```python
from build123d import *

# Parameters (mm, degrees)
CROQUIS1_W                = 7
CROQUIS1_H                = 18
SALIENTE_EXTRUIR1_DEPTH   = 9
SALIENTE_EXTRUIR1_2_DEPTH = 9
SALIENTE_EXTRUIR1_3_DEPTH = 9
SALIENTE_EXTRUIR1_4_DEPTH = 9
SALIENTE_EXTRUIR1_5_DEPTH = 9
SALIENTE_EXTRUIR1_6_DEPTH = 9
CROQUIS2_W                = 48.25
CROQUIS2_H                = 4
SALIENTE_EXTRUIR2_DEPTH   = 9
CROQUIS3_R                = 2.5
CROQUIS3_R_2              = 2
SALIENTE_EXTRUIR3_DEPTH   = 5.5
CROQUIS4_R                = 1
CORTAR_EXTRUIR1_DEPTH     = 53.278700252
CROQUIS5_W                = 6
CROQUIS5_H                = 8
CORTAR_EXTRUIR2_DEPTH     = 54.500584109


with BuildPart() as part:
    # Croquis1 → Saliente-Extruir1 (new body)
    with BuildSketch(Plane.XY):
        with Locations((11.75, 9)):
            Rectangle(CROQUIS1_W, CROQUIS1_H)
    extrude(amount=SALIENTE_EXTRUIR1_DEPTH)



with BuildPart() as body_2:
    # Croquis1 → Saliente-Extruir1 2 (new body)
    with BuildSketch(Plane.XY):
        with Locations((3.5, 9)):
            Rectangle(CROQUIS1_W, CROQUIS1_H)
    extrude(amount=SALIENTE_EXTRUIR1_2_DEPTH)


with BuildPart() as body_3:
    # Croquis1 → Saliente-Extruir1 3 (new body)
    with BuildSketch(Plane.XY):
        with Locations((20, 9)):
            Rectangle(CROQUIS1_W, CROQUIS1_H)
    extrude(amount=SALIENTE_EXTRUIR1_3_DEPTH)


with BuildPart() as body_4:
    # Croquis1 → Saliente-Extruir1 4 (new body)
    with BuildSketch(Plane.XY):
        with Locations((28.25, 9)):
            Rectangle(CROQUIS1_W, CROQUIS1_H)
    extrude(amount=SALIENTE_EXTRUIR1_4_DEPTH)


with BuildPart() as body_5:
    # Croquis1 → Saliente-Extruir1 5 (new body)
    with BuildSketch(Plane.XY):
        with Locations((36.5, 9)):
            Rectangle(CROQUIS1_W, CROQUIS1_H)
    extrude(amount=SALIENTE_EXTRUIR1_5_DEPTH)


with BuildPart() as body_6:
    # Croquis1 → Saliente-Extruir1 6 (new body)
    with BuildSketch(Plane.XY):
        with Locations((44.75, 9)):
            Rectangle(CROQUIS1_W, CROQUIS1_H)
    extrude(amount=SALIENTE_EXTRUIR1_6_DEPTH)


with BuildPart() as part_1:
    add(part.part)

    add(body_2.part)  # Saliente-Extruir2 merges body 2

    add(body_3.part)  # Saliente-Extruir2 merges body 3

    add(body_4.part)  # Saliente-Extruir2 merges body 4

    add(body_5.part)  # Saliente-Extruir2 merges body 5

    add(body_6.part)  # Saliente-Extruir2 merges body 6
    # Croquis2 → Saliente-Extruir2 (add)
    with BuildSketch(Plane.XY):
        with Locations((24.125, 9)):
            Rectangle(CROQUIS2_W, CROQUIS2_H)
    extrude(amount=SALIENTE_EXTRUIR2_DEPTH)

    # Croquis3 → Saliente-Extruir3 (add)
    # profile 1 of 12: a face of its own
    with BuildSketch(Plane.XY.offset(9)):
        with Locations(Location((3.5, 12, 0), (0, 0, 180))):
            Circle(CROQUIS3_R)
        with Locations((3.5, 12)):
            Circle(CROQUIS3_R_2, mode=Mode.SUBTRACT)
    # profile 2 of 12: a face of its own
    with BuildSketch(Plane.XY.offset(9)):
        with Locations(Location((11.75, 12, 0), (0, 0, 180))):
            Circle(CROQUIS3_R)
        with Locations((11.75, 12)):
            Circle(CROQUIS3_R_2, mode=Mode.SUBTRACT)
    # profile 3 of 12: a face of its own
    with BuildSketch(Plane.XY.offset(9)):
        with Locations(Location((20, 12, 0), (0, 0, 180))):
            Circle(CROQUIS3_R)
        with Locations((20, 12)):
            Circle(CROQUIS3_R_2, mode=Mode.SUBTRACT)
    # profile 4 of 12: a face of its own
    with BuildSketch(Plane.XY.offset(9)):
        with Locations(Location((28.25, 12, 0), (0, 0, 180))):
            Circle(CROQUIS3_R)
        with Locations((28.25, 12)):
            Circle(CROQUIS3_R_2, mode=Mode.SUBTRACT)
    # profile 5 of 12: a face of its own
    with BuildSketch(Plane.XY.offset(9)):
        with Locations(Location((36.5, 12, 0), (0, 0, 180))):
            Circle(CROQUIS3_R)
        with Locations((36.5, 12)):
            Circle(CROQUIS3_R_2, mode=Mode.SUBTRACT)
    # profile 6 of 12: a face of its own
    with BuildSketch(Plane.XY.offset(9)):
        with Locations(Location((44.75, 12, 0), (0, 0, 180))):
            Circle(CROQUIS3_R)
        with Locations((44.75, 12)):
            Circle(CROQUIS3_R_2, mode=Mode.SUBTRACT)
    # profile 7 of 12: a face of its own
    with BuildSketch(Plane.XY.offset(9)):
        with Locations(Location((11.75, 6, 0), (0, 0, 180))):
            Circle(CROQUIS3_R)
        with Locations((11.75, 6)):
            Circle(CROQUIS3_R_2, mode=Mode.SUBTRACT)
    # profile 8 of 12: a face of its own
    with BuildSketch(Plane.XY.offset(9)):
        with Locations(Location((20, 6, 0), (0, 0, 180))):
            Circle(CROQUIS3_R)
        with Locations((20, 6)):
            Circle(CROQUIS3_R_2, mode=Mode.SUBTRACT)
    # profile 9 of 12: a face of its own
    with BuildSketch(Plane.XY.offset(9)):
        with Locations(Location((28.25, 6, 0), (0, 0, 180))):
            Circle(CROQUIS3_R)
        with Locations((28.25, 6)):
            Circle(CROQUIS3_R_2, mode=Mode.SUBTRACT)
    # profile 10 of 12: a face of its own
    with BuildSketch(Plane.XY.offset(9)):
        with Locations(Location((36.5, 6, 0), (0, 0, 180))):
            Circle(CROQUIS3_R)
        with Locations((36.5, 6)):
            Circle(CROQUIS3_R_2, mode=Mode.SUBTRACT)
    # profile 11 of 12: a face of its own
    with BuildSketch(Plane.XY.offset(9)):
        with Locations(Location((44.75, 6, 0), (0, 0, 180))):
            Circle(CROQUIS3_R)
        with Locations((44.75, 6)):
            Circle(CROQUIS3_R_2, mode=Mode.SUBTRACT)
    # profile 12 of 12: a face of its own
    with BuildSketch(Plane.XY.offset(9)):
        with Locations(Location((3.5, 6, 0), (0, 0, 180))):
            Circle(CROQUIS3_R)
        with Locations((3.5, 6)):
            Circle(CROQUIS3_R_2, mode=Mode.SUBTRACT)
    extrude(amount=SALIENTE_EXTRUIR3_DEPTH)

    # Croquis4 → Cortar-Extruir1 (cut, through all)
    with BuildSketch(Plane.XY.offset(9)):
        with Locations((7.625, 9)):
            Circle(CROQUIS4_R)
        with Locations((15.875, 9)):
            Circle(CROQUIS4_R)
        with Locations((24.125, 9)):
            Circle(CROQUIS4_R)
        with Locations((32.375, 9)):
            Circle(CROQUIS4_R)
        with Locations((40.625, 9)):
            Circle(CROQUIS4_R)
    extrude(amount=-CORTAR_EXTRUIR1_DEPTH, mode=Mode.SUBTRACT)

    # Croquis5 → Cortar-Extruir2 (cut, through all)
    with BuildSketch(Plane.XZ):
        with Locations((3.5, 4.5)):
            Rectangle(CROQUIS5_W, CROQUIS5_H)
        with Locations((11.75, 4.5)):
            Rectangle(CROQUIS5_W, CROQUIS5_H)
        with Locations((20, 4.5)):
            Rectangle(CROQUIS5_W, CROQUIS5_H)
        with Locations((28.25, 4.5)):
            Rectangle(CROQUIS5_W, CROQUIS5_H)
        with Locations((36.5, 4.5)):
            Rectangle(CROQUIS5_W, CROQUIS5_H)
        with Locations((44.75, 4.5)):
            Rectangle(CROQUIS5_W, CROQUIS5_H)
    extrude(amount=-CORTAR_EXTRUIR2_DEPTH, mode=Mode.SUBTRACT)


solid = part_1.part
```
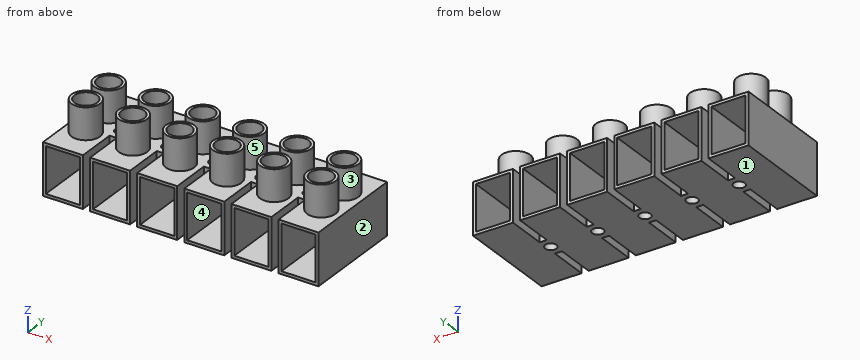
Read the model definition and answer for the solid it produces. Units are mm, in the model's axes. Face numbers are marked on the shaded views. A direction names the side the tool comes from. Give positions to 0.01 mm unless a question says otherwise; leave off trailing zeros. Write each loop counter-clockwise with the first axis right and the second up, starting at its lowest first coordinate (ties: lowest second). Pieces come first, ordered by that corner, then holes. Notation, with made-up numbers: (2, 86.25) -> (58, 86.25) arc R19 cw to (58, 109.25) -> close; hole circle Ø10 at (50, -37.5). An arc over 180 degrees is marked (long way). Answer in a Markdown table with one row per item.
1) Section A-A on x = 28.25 is taken. Give the vertices of the cut face in (y, z).
Results list:
| item | result |
|---|---|
| outline | (0, 0) -> (18, 0) -> (18, 0.5) -> (0, 0.5) -> close; (0, 8.5) -> (18, 8.5) -> (18, 9) -> (14.5, 9) -> (14.5, 14.5) -> (14, 14.5) -> (14, 9) -> (10, 9) -> (10, 14.5) -> (9.5, 14.5) -> (9.5, 9) -> (8.5, 9) -> (8.5, 14.5) -> (8, 14.5) -> (8, 9) -> (4, 9) -> (4, 14.5) -> (3.5, 14.5) -> (3.5, 9) -> (0, 9) -> close |
2) Section D-D on x = 5 is taken. Give the vertices of the cut face in (y, z).
Results list:
| item | result |
|---|---|
| outline | (0, 0) -> (18, 0) -> (18, 0.5) -> (0, 0.5) -> close; (0, 8.5) -> (18, 8.5) -> (18, 9) -> (14, 9) -> (14, 14.5) -> (13.32, 14.5) -> (13.32, 9) -> (10.68, 9) -> (10.68, 14.5) -> (10, 14.5) -> (10, 9) -> (8, 9) -> (8, 14.5) -> (7.32, 14.5) -> (7.32, 9) -> (4.68, 9) -> (4.68, 14.5) -> (4, 14.5) -> (4, 9) -> (0, 9) -> close |
3) A tool of negligible diameter and unlimited length cuts with its end or side. For the marked faces 4 and 5, from which of +Z, -Z, +X, -X, +Y, -Y can it reach the whole face along a straight path? Write none if from no direction.
Results list:
| item | result |
|---|---|
| face 4 | +Y, -Y |
| face 5 | +Z |
4) Section B-B on z = 2 is taken. Count the separate pieces of the cut face and the enclosed holes in it, plus the area to 3 significant figures.
Results list:
| item | result |
|---|---|
| separate pieces | 7 |
| enclosed holes | 5 |
| area | 117 mm^2 |
5) This flat-tipped pin is pushed along its axis until it touches: pin 1 Ø2.5 at (x, y) = (40.625, 9) entering from +Z. Where does it stop, or does it pass through?
Results list:
| item | result |
|---|---|
| pin 1 | z = 9 |
6) Straight lines are drawn through the part: line 1 (Y direction, x = 11.75, z = 13.2); line 2 (Z direction, x = 44.5, y = 7.25); line 3 (Y direction, x = 24, z = 5). For each, find the intervals that lie inside material, in ascending order. Write a range as [from, to].
Results list:
| item | result |
|---|---|
| line 1 | [3.5, 4], [8, 8.5], [9.5, 10], [14, 14.5] |
| line 2 | [0, 0.5], [8.5, 9] |
| line 3 | [7, 8.01], [9.99, 11] |
7) Determine the mould class of the marked faces 1, 2 and 3 for opening direction X: released by +X, released by -X, zero draft, split by the parting line, or undercut.
Results list:
| item | result |
|---|---|
| face 1 | zero draft |
| face 2 | released by +X |
| face 3 | undercut |
